Autodesk Inventor part; units mm, degrees
ref_plane "Work Plane1" through (36, 8.1705, 0) normal (1, 0, 0) x (0, 1, 0)
ref_plane "XZ Plane" through (0, 0, 0) normal (0, 1, 0) x (-1, 0, 0)
ref_plane "XY Plane" through (0, 0, 0) normal (0, 0, 1) x (1, 0, 0)
sketch "Sketch2" plane through (0, 0, 0) normal (0, 0, 1) x (1, 0, 0)
  line L0 (-8, 0.1705) -> (10, 0.1705)
  line L1 (36, 8.1705) -> (18, 8.1705)
  line L2 (14, 4.1705) -> (14, 4.1705)
  arc A0 (18, 8.1705) -> (14, 4.1705) centre (18, 4.1705) ccw
  arc A1 (10, 0.1705) -> (14, 4.1705) centre (10, 4.1705) ccw
  point P0 (14, 0.1705)
  point P1 (14, 8.1705)
  dimension "d9" = 44
  dimension "d15" = 8
  dimension "d16" = 22
  dimension "d17" = 22
  dimension "d24" = 4
ref_plane "Work Plane1" through (36, 8.1705, 0) normal (1, 0, 0) x (0, 1, 0)
sketch "Sketch3" plane through (36, 8.1705, 0) normal (1, 0, 0) x (0, 1, 0)
  line L0 (-1, 2) -> (-1, -2)
  line L1 (-1, -2) -> (1, -2)
  line L2 (1, -2) -> (1, 2)
  line L3 (1, 2) -> (-1, 2)
  line L4 (-1, 2) -> (1, -2) construction
  line L5 (-1, -2) -> (1, 2) construction
  point P0 (-8.1705, 0)
  point P1 (0, 0)
  dimension "d20" = 4
  dimension "d21" = 2
sweep "Sweep1" add profiles "Sketch3" path "Sketch2"
properties part number "SSSS"
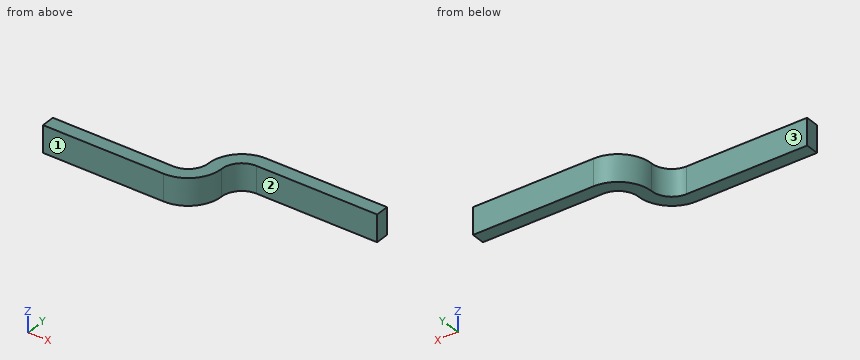
Can you work these out from the model? Positions are in its coordinate system, mm. Face numbers are marked on the shaded views. A direction names the side the tool comes from. Coordinates: 2 decimals unless noted, no trailing zeros. Loops run counter-clockwise (first coordinate to the right, second up) from the corner with the lowest first, then second, coordinate; pieces in that order, holes last. Notation, with made-up numbers: (66, 88) -> (122, 88) arc R12 ccw to (122, 111) -> close; hole circle Ø6 at (-3, 63). An arc over 180 degrees is marked (long way). Put each result on its own line as item: value. Start each with the question number.
Q1. I want a section at B-B (x = 23.5). Write out the boundary of the cut face in (y, z), plus the area to 3 significant figures.
Q2. I want a section at C-C (y = 6). Write out the boundary of the cut face in (x, z), plus the area to 3 significant figures.
Q3. If I drill on line 1 (Y direction, x = 23, z = 0.45); line 2 (Y direction, x = 8, z = -0.85); line 3 (X direction, y = 7.5, z = 1.25), over which ranges is the centre line in solid material (lowest first)? Write a range as [from, to].
Q4. I want a section at A-A (z = -1.35). Write out the boundary of the cut face in (x, y), plus the area to 3 significant figures.
Q5. For the marked faces 1, 2 and 3, which set-ups out of +Z, -Z, +X, -X, +Y, -Y let a thin tool reach every point of the face, with its end or its side?
Taken from the geometry:
1. outline: (7.17, -2) -> (9.17, -2) -> (9.17, 2) -> (7.17, 2) -> close
1. area: 8.00 mm2
2. outline: (13.35, -2) -> (15.62, -2) -> (15.62, 2) -> (13.35, 2) -> close
2. area: 9.10 mm2
3. line 1: y = [7.17, 9.17]
3. line 2: y = [-0.83, 1.17]
3. line 3: x = [14.27, 36]
4. outline: (-8, -0.83) -> (10, -0.83) arc R5 ccw to (15, 4.17) arc R3 cw to (18, 7.17) -> (36, 7.17) -> (36, 9.17) -> (18, 9.17) arc R5 ccw to (13, 4.17) arc R3 cw to (10, 1.17) -> (-8, 1.17) -> close
4. area: 97.1 mm2
5. face 1: +Z, -Z, +X, -X, -Y
5. face 2: +Z, -Z, +X, -Y
5. face 3: +Z, -Z, -X, +Y
